Check sheet for the drawn part. Datum: minimum x, y, z corner. Units: mm. Coordinates: 2 decimals unless noted, no trailing zeros. Write each loop counter-clockwise with the first axis right and the second up, starting at its lowest first coordinate (ties: lowest second). Pieces come first, ordered by that corner, then holes. Notation, with made-up numbers: M -13.75,86.5 L 41.25,86.5 A14 cw 41.25,113.5 Z; hole C -17.75,64.25 d6. An arc over 180 degrees is marked long. Answer as a JSON object with one key per item and string values. Group by question number.
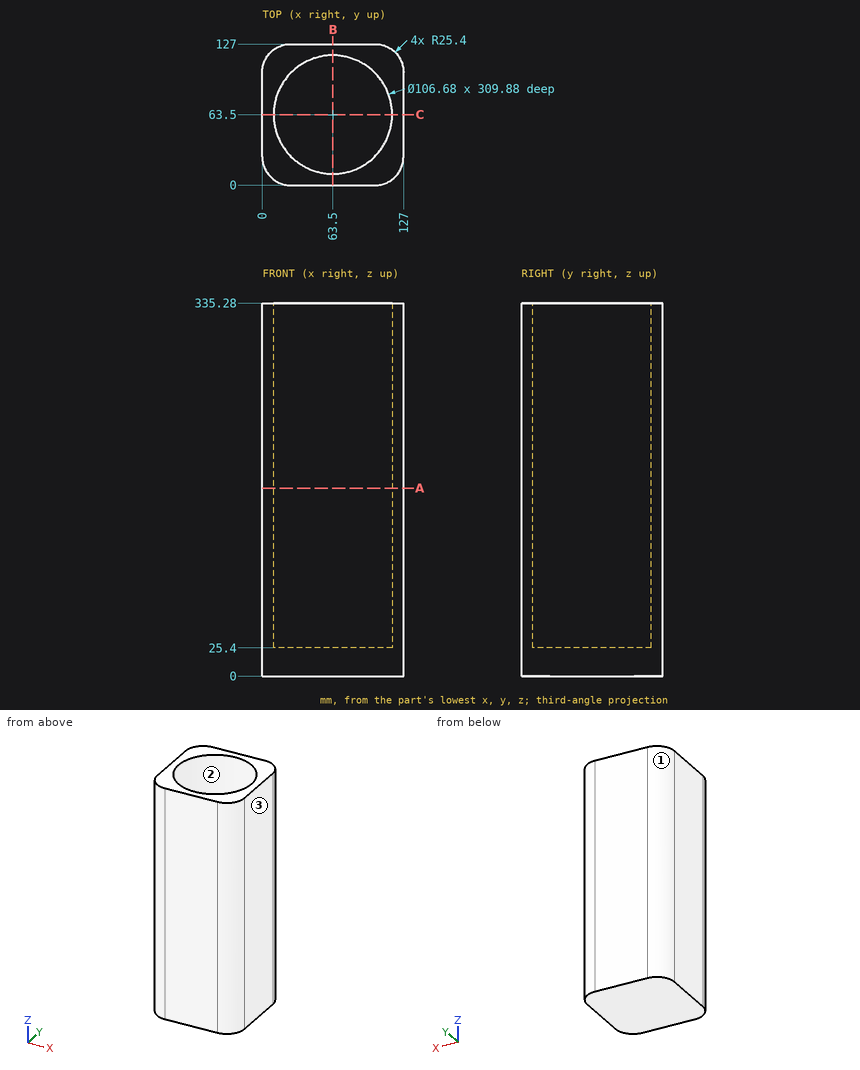
1) Section check B-B (x = 63.5). Record the cut outline in (y, z).
2) Material ranges on probe 1 along Y at (x, z) = (63.5, 109); probe 2 along X at (y, z) = (65, 123.5); probe 3 along Z at (x, y) = (83, 38.5), recorded low to high. Write a range as [from, to].
3) Section check A-A (z = 169). Record the cut outline in (x, y), then the cut area to 3 significant figures.
4) Go/stop test with flat-tipped pins: pin 1 Ø3 at (x, y) = (27.5, 60.5) entering from -Z; pin 2 Ø1 at (x, z) = (114, 45) entering from +Y. Record where each tip stops, or that it passes through.
5) Draft check along X on the marked faces 1, 2 and 3. Enter one of: +X half, -X half, draft (parallel to the pull), parting line (faces both ways), or undercut.
Entries:
{
 "1": {"outline": "M 0,0 L 127,0 L 127,335.28 L 116.84,335.28 L 116.84,25.4 L 10.16,25.4 L 10.16,335.28 L 0,335.28 Z"},
 "2": {"probe 1": "[0, 10.16], [116.84, 127]", "probe 2": "[0, 10.18], [116.82, 127]", "probe 3": "[0, 25.4]"},
 "3": {"outline": "M 0,25.4 A25.4 ccw 25.4,0 L 101.6,0 A25.4 ccw 127,25.4 L 127,101.6 A25.4 ccw 101.6,127 L 25.4,127 A25.4 ccw 0,101.6 Z; hole C 63.5,63.5 d106.68", "area": "6,640 mm^2"},
 "4": {"pin 1": "z = 0", "pin 2": "y = 124.04"},
 "5": {"face 1": "-X half", "face 2": "undercut", "face 3": "+X half"}
}
